Geometry: final body of the model. Coordinates: model frame, mm. Face numbers are marked on the shaded views. A direction names the side the tool comes from. Round coordinates to 2 decimals unless told otherwise and drop trailing zeros. Loops run counter-clockwise (first coordinate to the right, second up) from the corner with the lowest first, then second, coordinate; pieces in that order, holes last. Notation, with made-up numbers: (75, 27.5) - (126, 27.5) arc R32 cw to (126, 57.5) - close; hole circle Ø8 at (43, 67). An arc over 180 degrees is marked (long way). Return JSON: item names as keys, results as strings. Group by question number.
1. Section A-A on y = 0. Return loops of the section in (x, z).
2. Material intervals for probe 1 along X at (y, z) = (0, -9.1); probe 2 along Y at (x, z) = (-8, -1.25); probe 3 along Y at (x, z) = (0, -6.95), sorted ascending.
3. Section D-D on x = -7.5. Return loops of the section in (y, z).
4. First-contact query: pin 1 Ø1.2 at (x, y) = (-4.5, -0.5) entering from +Z; pin 2 Ø5.5 at (x, y) = (0, 0) entering from -Z. Flat tips, straight axial feed; report the tip coordinate or a pass-through.
5. Draft query along Y for the marked faces 1, 2, 3 and 4. Return one class per face: +Y half, -Y half, draft (parallel to the pull), parting line (faces both ways), or undercut.
6. Section B-B on x = 0. Return loops of the section in (y, z), and give its area (3 significant figures).
7. Section C-C on z = -0.75. Return loops of the section in (x, y).
8. Set-up query: the marked faces 5 and 6. Return all of +Z, -Z, +X, -X, +Y, -Y with unobstructed straight access to the full face (end or side cutting, diameter ignored); none if empty.
from build123d import *

# Parameters (mm, degrees)
SKETCH_W         = 20
SKETCH_H         = 40
PAD_DEPTH        = 10
HOLE_D           = 6
HOLE_CSINK_D     = 13
HOLE_CSINK_ANGLE = 60
SKETCH002_W      = 20
SKETCH002_H      = 4
POCKET_DEPTH     = 8


with BuildPart() as part:
    # Sketch → Pad (new body)
    with BuildSketch(Plane.XY):
        Rectangle(SKETCH_W, SKETCH_H)
    extrude(amount=-PAD_DEPTH)

    # Hole (through all)
    with Locations(Plane.XY):
        with Locations((0, 0)):
            CounterSinkHole(HOLE_D / 2, HOLE_CSINK_D / 2, counter_sink_angle=HOLE_CSINK_ANGLE)

    # Sketch002 (on Face4 of Hole) → Pocket (cut)
    with BuildSketch(Plane.XY):
        Rectangle(SKETCH002_W, SKETCH002_H)
    extrude(amount=-POCKET_DEPTH, mode=Mode.SUBTRACT)


solid = part.part
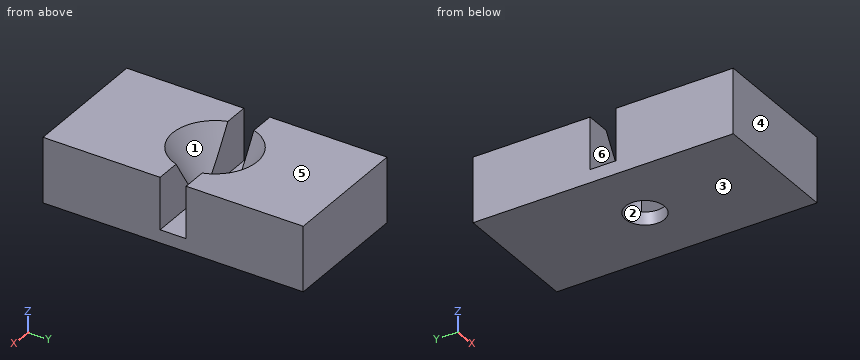
Taken from the geometry:
{
 "1": {"outline": "(-10, -10) - (-3, -10) - (-3, -8) - (-10, -8) - close; (3, -10) - (10, -10) - (10, -8) - (3, -8) - close"},
 "2": {"probe 1": "-10 to -3, 3 to 10", "probe 2": "-20 to -2, 2 to 20", "probe 3": "-20 to -3, 3 to 20"},
 "3": {"outline": "(-20, -10) - (20, -10) - (20, 0) - (2, 0) - (2, -8) - (-2, -8) - (-2, 0) - (-20, 0) - close"},
 "4": {"pin 1": "z = -8", "pin 2": "through"},
 "5": {"face 1": "undercut", "face 2": "undercut", "face 3": "draft", "face 4": "-Y half"},
 "6": {"outline": "(-20, -10) - (-3, -10) - (-3, -6.06) - (-6.5, 0) - (-20, 0) - close; (3, -10) - (20, -10) - (20, 0) - (6.5, 0) - (3, -6.06) - close", "area": "319 mm2"},
 "7": {"outline": "(-10, -20) - (10, -20) - (10, -2) - (5.73, -2) arc R6.07 cw to (-5.73, -2) - (-10, -2) - close; (-10, 2) - (-5.73, 2) arc R6.07 cw to (5.73, 2) - (10, 2) - (10, 20) - (-10, 20) - close"},
 "8": {"face 5": "+Z, +X, -X, +Y, -Y", "face 6": "+Z, +X, -X"}
}
